from build123d import *

# Parameters (mm, degrees)
F0_R     = 7.5
F1_DEPTH = 3.2
F2_SIZE2 = 7
F2_SIZE  = 9
F3_SIZE  = 5


with BuildPart() as f1:
    # F0 (on Top) → F1 (new body)
    with BuildSketch(Plane.XY):
        Polygon((-16, 0), (-16, -24), (16, -24), (16, 0), (11, 2), (11, 6), (15, 8), (15, 19), (-15, 19), (-15, 8), (-11, 6), (-11, 2), align=None)
        with Locations((0, -7.5)):
            Circle(F0_R, mode=Mode.SUBTRACT)
    extrude(amount=F1_DEPTH)

    # F2
    f2_edges = [f1.edges().sort_by_distance(p)[0] for p in [
        (-16, -24, 1.6),
        (16, -24, 1.6),
    ]]
    f2_side = f1.faces().sort_by_distance((0, -24, 1.6))[0]
    chamfer(f2_edges, length=F2_SIZE, length2=F2_SIZE2, reference=f2_side)

    # F3
    f3_edges = [f1.edges().sort_by_distance(p)[0] for p in [
        (-15, 19, 1.6),
        (15, 19, 1.6),
    ]]
    chamfer(f3_edges, length=F3_SIZE)


solid = f1.part
Model file for the job. Use its own axes, mm. A direction names the side the tool comes from. Give positions to 0.01 mm unless a question says otherwise; leave off trailing zeros. Order: outer loops, then holes, each group sorted by start corner. A loop starts at its lowest first (then second) coordinate and runs counter-clockwise, first axis right, second up. Notation, with made-up numbers: (10, -10.5) - (33, -10.5) arc R27 cw to (33, 20.5) - close; hole circle Ø7 at (-7.5, 76.5). An arc over 180 degrees is marked (long way). Write item = value, one per line. Start each with the question number.
1. Cut at C-C, the plane z = 0.85. List the corners of the cut face in (x, y), and give its area (3 significant figures).
2. Which spindle directions (+Z, -Z, +X, -X, +Y, -Y) get a long thin tool onto all of the face, cutting with end or side? Do faces 1 (the flat face through (-15, 11, 2)), 2 (the flat face through (13, 7, 2)), 3 (the flat face through (-11, 4, 2)). Say none if no direction does.
3. Drop flat-ended pins along their axis: P1, Ø12, axis at x = 0, y = -7.5, coming from the -Z side; P2, Ø1.6, axis at y = 12, z = 2, coming from the -X side. Give the stop position or say it passes through.
4. Cut at B-B, the plane y = -7.5. List the corners of the cut face in (x, z).
5. Probe line 1 along Y through (x, z) = (0, 0.8); line 2 along X through (y, z) = (-4, 2.85); line 3 along Y through (x, z) = (12, 1.4). List the from-to ranges inside material, lowest first.
6. Two-plate mould, pull along X, no slides. Class faces 4 (the flat face through (0, -24, 2)), 5 (the flat face through (16, -9, 2)), 6 (the flat face through (-13.5, 1, 1.6)), 7 (the cylindrical face through (-0.976, -0.064, 1.578)): pulls with the +X half, pulls with the -X half, needs draft (parallel to the pull), parting line crosses it, or undercut.
7. Cut at D-D, the plane y = 11. List the corners of the cut face in (x, z), and give its area (3 significant figures).
8. Cut at A-A, the plane x = 0. List the corners of the cut face in (y, z), and give its area (3 significant figures).
Taken from the geometry:
q1.outline = (-16, -17) - (-7, -24) - (7, -24) - (16, -17) - (16, 0) - (11, 2) - (11, 6) - (15, 8) - (15, 14) - (10, 19) - (-10, 19) - (-15, 14) - (-15, 8) - (-11, 6) - (-11, 2) - (-16, 0) - close; hole circle Ø15 at (0, -7.5)
q1.area = 1,030 mm²
q2.face_1 = +Z, -Z, -X, +Y
q2.face_2 = +Z, -Z, +X
q2.face_3 = +Z, -Z, -X
q3.P1 = through
q3.P2 = -15
q4.outline = (-16, 0) - (-7.5, 0) - (-7.5, 3.2) - (-16, 3.2) - close; (7.5, 0) - (16, 0) - (16, 3.2) - (7.5, 3.2) - close
q5.line_1 = -24 to -15, 0 to 19
q5.line_2 = -16 to -6.63, 6.63 to 16
q5.line_3 = -20.11 to 1.6, 6.5 to 17
q6.face_4 = needs draft
q6.face_5 = pulls with the +X half
q6.face_6 = pulls with the -X half
q6.face_7 = undercut
q7.outline = (-15, 0) - (15, 0) - (15, 3.2) - (-15, 3.2) - close
q7.area = 96.0 mm²
q8.outline = (-24, 0) - (-15, 0) - (-15, 3.2) - (-24, 3.2) - close; (0, 0) - (19, 0) - (19, 3.2) - (0, 3.2) - close
q8.area = 89.6 mm²
